```python
from build123d import *

# Parameters (mm, degrees)
SKETCH_1_R             = 1.55
EXTRUDE_397_DEPTH      = 2.5
EXTRUDE_START          = 2.5
EXTRUDE_640_DEPTH      = 7.5
SKETCH_3_W             = 4.5
SKETCH_3_H             = 12.978713764
EXTRUDE_1_DEPTH        = 9.75
CHAMFER_1_SIZE         = 1
CUT_EXTRUDE_1239_DEPTH = 2
CUT_EXTRUDE_M3_REACH   = 27.038
SKETCH_6_R             = 1.55
FILLET_5_R             = 0.75
FILLET_6_R             = 0.25


with BuildPart() as part:
    # 草图1 → Extrude 397 (new body)
    with BuildSketch(Plane(origin=(0, 0, 0), x_dir=(1, 0, 0), z_dir=(0, 1, 0))):
        with BuildLine():
            Line((10.1243866, 13.845154317), (-6.15423406, 2.01804411))
            ThreePointArc((-6.15423406, 2.01804411), (-7.315700706, -5.315167685), (0.017511089, -6.476634331))
            Line((0.017511089, -6.476634331), (10.1243866, 0.866440553))
            Line((10.1243866, 0.866440553), (10.1243866, 13.845154317))
        make_face()
        with Locations(Location((0, 0, 0), (0, 0, 270))):
            Circle(SKETCH_1_R, mode=Mode.SUBTRACT)
    extrude(amount=EXTRUDE_397_DEPTH)

    # 草图2 → Extrude 640 (add)
    with BuildSketch(Plane(origin=(0, 0, 0), x_dir=(1, 0, 0), z_dir=(0, 1, 0)).offset(EXTRUDE_START)):
        Polygon((0.017511089, -6.476634331), (1.193081594, -8.09466832), (11.299957105, -0.751593436), (10.1243866, 0.866440553), align=None)
        Polygon((-7.329804565, 3.636078099), (0.809505765, 9.549633202), (1.98507627, 7.931599213), (-6.15423406, 2.01804411), align=None)
    extrude(amount=-EXTRUDE_640_DEPTH)

    # 草图3 → 限位-1 (add)
    with BuildSketch(Plane(origin=(0, 0, 0), x_dir=(1, 0, 0), z_dir=(0, 1, 0))):
        with Locations((12.3743866, 7.355797435)):
            Rectangle(SKETCH_3_W, SKETCH_3_H)
    extrude(amount=EXTRUDE_1_DEPTH)

    # 倒角1
    chamfer_1_edges = [part.edges().sort_by_distance(p)[0] for p in [
        (0, 2.5, -1.55),
    ]]
    chamfer(chamfer_1_edges, length=CHAMFER_1_SIZE)

    # 草图5 → Cut-Extrude 1239 (cut)
    with BuildSketch(Plane.ZY.offset(-10.1243866)):
        Polygon((-4.151503441, 5.755), (-5.753650438, 8.53), (-8.957944432, 8.53), (-10.560091429, 5.755), (-8.957944432, 2.98), (-5.753650438, 2.98), align=None)
    extrude(amount=-CUT_EXTRUDE_1239_DEPTH, mode=Mode.SUBTRACT)

    # 草图6 → M3螺孔 (cut, up to next)
    with BuildSketch(Plane.ZY.offset(-10.1243866), mode=Mode.PRIVATE) as cut_extrude_m3_sk1:
        with Locations((-7.355797435, 5.755)):
            Circle(SKETCH_6_R)
    cut_extrude_m3_tool1 = extrude(cut_extrude_m3_sk1.sketch, amount=-CUT_EXTRUDE_M3_REACH, mode=Mode.PRIVATE) & part.part
    add(cut_extrude_m3_tool1.solids().sort_by_distance((10.124387, 5.755, -7.355797))[0], mode=Mode.SUBTRACT)

    # 圆角5
    fillet_5_edges = [part.edges().sort_by_distance(p)[0] for p in [
        (11.299957105, -1.25, 0.751593436),
        (1.193081594, -1.25, 8.09466832),
        (1.98507627, 1.25, -7.931599213),
        (-7.329804565, -1.25, -3.636078099),
        (0.809505765, -1.25, -9.549633202),
        (-6.15423406, 1.25, -2.01804411),
        (0.017511089, 1.25, 6.476634331),
    ]]
    fillet(fillet_5_edges, radius=FILLET_5_R)

    # 圆角6
    fillet_6_edges = [part.edges().sort_by_distance(p)[0] for p in [
        (10.1243866, 1.25, -0.866440553),
    ]]
    fillet(fillet_6_edges, radius=FILLET_6_R)


solid = part.part
```
Source: CAD feature listing. Evaluate the final solid. Frame: model axes, mm. A direction names the side the tool comes from. Round coordinates to 2 decimals unless told otherwise and drop trailing zeros. Loops run counter-clockwise (first coordinate to the right, second up) from the corner with the lowest first, then second, coordinate; pieces in that order, holes last.
(1) Access query for faces 5 (the flat face through (3, 0, -3)), 6 (the flat face through (-2.028, -2.465, -5.016)), 7 (the flat face through (11.11, 4.39, -9.77)), 8 (the flat face through (5.142, -2.465, 2.754)), 9 (the flat face through (10.124, 7, -4)). Directions: +Z, -Z, +X, -X, +Y, -Y. A direction counts if a zero-diameter tool reaches every point of the face in a straight line with its end or side. Return the directions, or none.
From the geometry:
face 5: -Y
face 6: +X, -Y
face 7: -X
face 8: -X, -Y
face 9: +Z, -Z, -X, +Y
(2) Section query B-B (y = 8.25). Output: boundary loops of the cut face in (x, z), and give its area (3 significant figures).
From the geometry:
outline: (10.12, -13.85) - (14.62, -13.85) - (14.62, -0.87) - (10.12, -0.87) - (10.12, -5.59) - (12.12, -5.59) - (12.12, -9.12) - (10.12, -9.12) - close
area: 51.3 mm2
(3) Material intervals for probe 1 along Y at (x, z) = (-5.5, -2); probe 2 along X at (y, z) = (4, -3.75); probe 3 along Y at (x, z) = (0.5, -9), sorted ascending.
From the geometry:
probe 1: y = 0 to 2.5
probe 2: x = 10.12 to 14.62
probe 3: y = -5 to 2.5
(4) Section query A-A (y = -4). Output: boundary loops of the cut face in (x, z), and give its area (3 significant figures).
From the geometry:
outline: (-6.89, -3.03) arc R0.75 ccw to (-6.72, -4.08) - (0.2, -9.11) arc R0.75 ccw to (1.25, -8.94) - (1.99, -7.93) - (-6.15, -2.02) - close; (0.02, 6.48) - (10.12, -0.87) - (10.86, 0.14) arc R0.75 ccw to (10.69, 1.19) - (1.8, 7.65) arc R0.75 ccw to (0.75, 7.49) - close
area: 44.6 mm2
(5) Pull-direction query (X, two-part tool) for faces 1 (the cylindrical face through (1.234, -1.303, 7.786)), 2 (the flat face through (1.613, -2.031, -8.444)), 3 (the flat face through (12, 9.75, -7)), 4 (the flat face through (10.5, -1.2, -0.35)); classes: +X half, -X half, draft (parallel to the pull), parting line (faces both ways), or undercut.
From the geometry:
face 1: parting line
face 2: undercut
face 3: draft
face 4: +X half
(6) Section query C-C (x = 5.75). Output: boundary loops of the cut face in (y, z), and give its area (3 significant figures).
From the geometry:
outline: (-5, 2.31) - (0, 2.31) - (0, -10.67) - (2.5, -10.67) - (2.5, 4.78) - (-5, 4.78) - close
area: 51.0 mm2
(7) Contact query for flat-ended pins moving along their axis: pin 1 Ø2 at (x, z) = (11, -7) entering from -Y; pin 2 Ø1 at (y, z) = (-2.5, 2.5) entering from +X; pin 3 Ø6 at (y, z) = (6.5, -9) entering from -X; pin 4 Ø3 at (y, z) = (5.5, 0) entering from +X. Output: stop coordinate, or through.
From the geometry:
pin 1: stops at y = 0
pin 2: stops at x = 9.58
pin 3: stops at x = 10.12
pin 4: stops at x = 14.62
